Here's how the part is built. I have some questions about the finished solid (model axes, mm). Face numbers are marked on the shaded views. A direction names the side the tool comes from. Round coordinates to 2 decimals unless told otherwise and drop trailing zeros. Write each loop counter-clockwise with the first axis right and the second up, starting at its lowest first coordinate (ties: lowest second). Pieces come first, ordered by that corner, then holes. Notation, with made-up numbers: M -15.75,75.25 L 33.25,75.25 A27 cw 33.25,94.25 Z; hole C 88.25,49.25 d9. An arc over 180 degrees is marked long. Write item = value, one per line. Start each with the question number.
(1) I want a section at B-B (x = 58). List the corners of the cut face in (y, z) for me, and give its area (3 significant figures).
(2) I need wall thicknesses on line 1 along X through (y, z) = (30.75, 21); line 2 along Z through (x, y) = (20.5, 6.5); line 3 along X through (y, z) = (10, 23.5). Which ranges of each line are inside material? Lowest first, please.
(3) I want a section at D-D (x = 83). Give the number of separate pieces and of enclosed holes in the cut face, and give its area (3 significant figures).
(4) Will these pins go through, and if not, where does the flat tip stop? pin 1 Ø1 at (y, z) = (1.5, -35) entering from -X; pin 2 Ø5.5 at (x, y) = (86.5, 2.5) entering from +Z; pin 3 Ø1.5 at (x, z) = (84, -24) entering from +Y; pin 4 Ø4 at (x, y) = (28, 17.5) entering from -Z.
(5) I want a section at C-C (y = 21.5). List the corners of the cut face in (x, z) for me, and give its area (3 significant figures).
(6) I want a section at A-A (y = 8.5). List the corners of the cut face in (x, z) for me, and give its area (3 significant figures).
(7) On a 3-axis mill with a long thin cutter (end or side, diameter ignored), from which of +Z, -Z, +X, -X, +Y, -Y can I reach the whole of each face in a straight line? I mean the marked faces 4, 5 and 6. Say none if no direction works.
(8) If we mould it in two halves opening along X, with no side actions, what happens to the marked faces 1, 2 and 3? For each: released by +X, released by -X, zero draft, split by the parting line, or undercut.
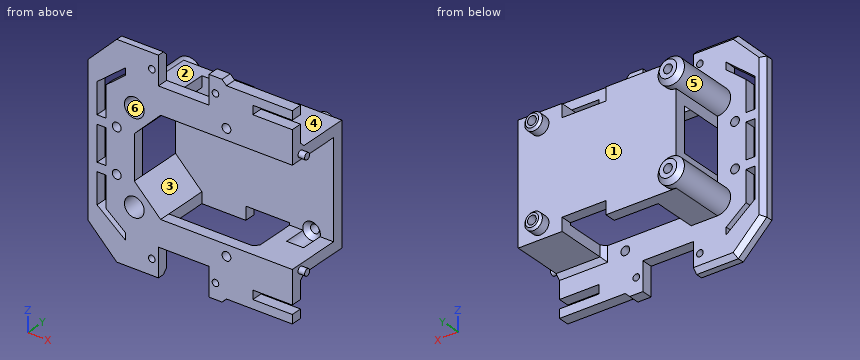
```python
from build123d import *

# Parameters (mm, degrees)
SKETCH1_R           = 2
SKETCH1_R_2         = 1.5
BOSS_EXTRUDE1_DEPTH = 5
SKETCH2_W           = 4
SKETCH2_H           = 16
CUT_EXTRUDE1_DEPTH  = 5
BOSS_EXTRUDE3_DEPTH = 25
SKETCH4_W           = 72
SKETCH4_H           = 54
BOSS_EXTRUDE4_DEPTH = 5
SKETCH5_W           = 40
SKETCH5_H           = 20
CUT_EXTRUDE2_DEPTH  = 123.576506721
SKETCH6_W           = 20
SKETCH6_H           = 6
CUT_EXTRUDE4_DEPTH  = 10
BOSS_EXTRUDE5_START = -5
SKETCH7_R           = 4
BOSS_EXTRUDE5_DEPTH = 5
SKETCH8_R           = 2
CUT_EXTRUDE5_DEPTH  = 10
CUT_EXTRUDE6_START  = 10
SKETCH9_R           = 4
CUT_EXTRUDE6_DEPTH  = 10
BOSS_EXTRUDE6_START = 5
SKETCH10_R          = 6
BOSS_EXTRUDE6_DEPTH = 30
SKETCH11_R          = 2
CUT_EXTRUDE7_DEPTH  = 10
CUT_EXTRUDE8_START  = 20
SKETCH12_R          = 4.5
CUT_EXTRUDE8_DEPTH  = 129.434311913
SKETCH14_R          = 4.5
CUT_EXTRUDE11_DEPTH = 108.158760724
SKETCH13_R          = 1.5
BOSS_EXTRUDE8_DEPTH = 3
CHAMFER2_SIZE       = 1
CHAMFER3_SIZE       = 2
CHAMFER4_SIZE       = 2
CHAMFER5_SIZE       = 2


with BuildPart() as part:
    # Sketch1 → Boss-Extrude1 (new body)
    with BuildSketch(Plane(origin=(0, 0, 0), x_dir=(1, 0, 0), z_dir=(0, 1, 0))):
        Polygon((0, 34), (0, -34), (13, -47), (32, -47), (32, -34), (55, -34), (55, -47), (61, -47), (63, -45), (93, -45), (93, -41), (75, -41), (75, -37), (93, -37), (93, -22), (33, -22), (21, -10), (21, 10), (33, 22), (93, 22), (93, 37), (75, 37), (75, 41), (93, 41), (93, 45), (63, 45), (61, 47), (55, 47), (55, 34), (32, 34), (32, 47), (13, 47), align=None)
        with Locations(Location((13, -10, 0), (0, 0, 270))):
            Circle(SKETCH1_R, mode=Mode.SUBTRACT)
        with Locations(Location((29, -40, 0), (0, 0, 270))):
            Circle(SKETCH1_R_2, mode=Mode.SUBTRACT)
        with Locations(Location((58, -40, 0), (0, 0, 270))):
            Circle(SKETCH1_R_2, mode=Mode.SUBTRACT)
        with Locations(Location((63, -27, 0), (0, 0, 270))):
            Circle(SKETCH1_R, mode=Mode.SUBTRACT)
        with Locations(Location((13, 10, 0), (0, 0, 90))):
            Circle(SKETCH1_R, mode=Mode.SUBTRACT)
        with Locations(Location((29, 40, 0), (0, 0, 90))):
            Circle(SKETCH1_R_2, mode=Mode.SUBTRACT)
        with Locations(Location((58, 40, 0), (0, 0, 90))):
            Circle(SKETCH1_R_2, mode=Mode.SUBTRACT)
        with Locations(Location((63, 27, 0), (0, 0, 90))):
            Circle(SKETCH1_R, mode=Mode.SUBTRACT)
    extrude(amount=BOSS_EXTRUDE1_DEPTH)

    # Sketch2 → Cut-Extrude1 (cut)
    with BuildSketch(Plane(origin=(0, 5, 0), x_dir=(1, 0, 0), z_dir=(0, 1, 0))):
        Polygon((17, 33.205766921), (17, 36.408329997), (4, 26), (4, 12), (8, 12), (8, 26), align=None)
        with Locations((6, 0)):
            Rectangle(SKETCH2_W, SKETCH2_H)
        Polygon((17, -33.205766921), (17, -36.408329997), (4, -26), (4, -12), (8, -12), (8, -26), align=None)
    extrude(amount=-CUT_EXTRUDE1_DEPTH, mode=Mode.SUBTRACT)

    # Sketch3 → Boss-Extrude3 (add)
    with BuildSketch(Plane(origin=(0, 5, 0), x_dir=(1, 0, 0), z_dir=(0, 1, 0))):
        Polygon((21, 27), (21, 10), (33, 22), (93, 22), (93, 27), align=None)
        Polygon((93, -27), (93, -22), (33, -22), (21, -10), (21, -27), align=None)
    extrude(amount=BOSS_EXTRUDE3_DEPTH)

    # Sketch4 → Boss-Extrude4 (add)
    with BuildSketch(Plane(origin=(0, 30, 0), x_dir=(1, 0, 0), z_dir=(0, 1, 0))):
        with Locations((57, 0)):
            Rectangle(SKETCH4_W, SKETCH4_H)
    extrude(amount=-BOSS_EXTRUDE4_DEPTH)

    # Sketch5 → Cut-Extrude2 (cut, through all)
    with BuildSketch(Plane.XY.offset(27)):
        with Locations((53, 15)):
            Rectangle(SKETCH5_W, SKETCH5_H)
    extrude(amount=-CUT_EXTRUDE2_DEPTH, mode=Mode.SUBTRACT)

    # Sketch6 → Cut-Extrude4 (cut)
    with BuildSketch(Plane(origin=(0, 30, 0), x_dir=(1, 0, 0), z_dir=(0, 1, 0))):
        with Locations((63, 24)):
            Rectangle(SKETCH6_W, SKETCH6_H)
        with Locations((63, -24)):
            Rectangle(SKETCH6_W, SKETCH6_H)
    extrude(amount=-CUT_EXTRUDE4_DEPTH, mode=Mode.SUBTRACT)

    # Sketch7 → Boss-Extrude5 (add)
    with BuildSketch(Plane.XZ.offset(-25).offset(BOSS_EXTRUDE5_START)):
        with Locations(Location((83, 21, 0), (0, 0, 270))):
            Circle(SKETCH7_R)
        with Locations(Location((83, -21, 0), (0, 0, 270))):
            Circle(SKETCH7_R)
    extrude(amount=-BOSS_EXTRUDE5_DEPTH)

    # Sketch8 → Cut-Extrude5 (cut)
    with BuildSketch(Plane(origin=(0, 35, 0), x_dir=(1, 0, 0), z_dir=(0, 1, 0))):
        with Locations(Location((83, 21, 0), (0, 0, 270))):
            Circle(SKETCH8_R)
    cut_extrude5 = extrude(amount=-CUT_EXTRUDE5_DEPTH, mode=Mode.SUBTRACT)

    # Sketch9 → Cut-Extrude6 (cut)
    with BuildSketch(Plane.XZ.offset(-25).offset(CUT_EXTRUDE6_START)):
        with Locations(Location((83, -21, 0), (0, 0, 270))):
            Circle(SKETCH9_R)
    cut_extrude6 = extrude(amount=-CUT_EXTRUDE6_DEPTH, mode=Mode.SUBTRACT)

    # Sketch10 → Boss-Extrude6 (add)
    with BuildSketch(Plane(origin=(0, 30, 0), x_dir=(1, 0, 0), z_dir=(0, 1, 0)).offset(BOSS_EXTRUDE6_START)):
        with Locations(Location((21, 21, 0), (0, 0, 270))):
            Circle(SKETCH10_R)
    boss_extrude6 = extrude(amount=-BOSS_EXTRUDE6_DEPTH)

    # Sketch11 → Cut-Extrude7 (cut)
    with BuildSketch(Plane(origin=(0, 35, 0), x_dir=(1, 0, 0), z_dir=(0, 1, 0))):
        with Locations(Location((21, 21, 0), (0, 0, 270))):
            Circle(SKETCH11_R)
    cut_extrude7 = extrude(amount=-CUT_EXTRUDE7_DEPTH, mode=Mode.SUBTRACT)

    # Sketch12 → Cut-Extrude8 (cut, through all)
    with BuildSketch(Plane(origin=(0, 5, 0), x_dir=(1, 0, 0), z_dir=(0, 1, 0)).offset(CUT_EXTRUDE8_START)):
        with Locations(Location((21, 21, 0), (0, 0, 270))):
            Circle(SKETCH12_R)
    extrude(amount=-CUT_EXTRUDE8_DEPTH, mode=Mode.SUBTRACT)

    # Mirror11: Cut-Extrude5, Cut-Extrude6 across plane
    add(cut_extrude5.mirror(Plane.XY), mode=Mode.SUBTRACT)
    add(cut_extrude6.mirror(Plane.XY), mode=Mode.SUBTRACT)

    # Mirror12: Boss-Extrude6 across plane
    add(boss_extrude6.mirror(Plane.XY))

    # Mirror16: Cut-Extrude7 across plane
    add(cut_extrude7.mirror(Plane.XY), mode=Mode.SUBTRACT)

    # Sketch14 → Cut-Extrude11 (cut, through all)
    with BuildSketch(Plane(origin=(0, 25, 0), x_dir=(1, 0, 0), z_dir=(0, 1, 0))):
        with Locations(Location((21, -21, 0), (0, 0, 270))):
            Circle(SKETCH14_R)
    extrude(amount=-CUT_EXTRUDE11_DEPTH, mode=Mode.SUBTRACT)

    # Sketch13 → Boss-Extrude8 (add)
    with BuildSketch(Plane(origin=(93, 0, 0), x_dir=(0, 0, -1), z_dir=(1, 0, 0))):
        with Locations(Location((24.5, 5, 0), (0, 0, 180))):
            Circle(SKETCH13_R)
    boss_extrude8 = extrude(amount=BOSS_EXTRUDE8_DEPTH)

    # Mirror19: Boss-Extrude8 across plane
    add(boss_extrude8.mirror(Plane.XY))

    # Chamfer2
    chamfer2_edges = [part.edges().sort_by_distance(p)[0] for p in [
        (83, 35, 25),
        (83, 35, -17),
    ]]
    chamfer(chamfer2_edges, length=CHAMFER2_SIZE)

    # Chamfer3
    chamfer3_edges = [part.edges().sort_by_distance(p)[0] for p in [
        (22.5, 5, -47),
        (6.5, 5, -40.5),
        (0, 5, 0),
        (6.5, 5, 40.5),
        (21, 35, -27),
        (21, 35, 27),
        (22.5, 5, 47),
    ]]
    chamfer(chamfer3_edges, length=CHAMFER3_SIZE)

    # Chamfer4
    chamfer4_edges = [part.edges().sort_by_distance(p)[0] for p in [
        (83, 5, -27),
        (83, 5, 27),
        (73, 5, 24.5),
        (73, 5, -24.5),
    ]]
    chamfer(chamfer4_edges, length=CHAMFER4_SIZE)

    # Chamfer5
    chamfer5_edges = [part.edges().sort_by_distance(p)[0] for p in [
        (83, 25, -23),
        (83, 25, 23),
    ]]
    chamfer(chamfer5_edges, length=CHAMFER5_SIZE - 0.0001)  # a hair under: the kernel refuses the full size


solid = part.part
```
Returned:
q1.outline = M 0,-47 L 5,-47 L 5,-41.5 L 0,-41.5 Z; M 0,-38.5 L 5,-38.5 L 5,-22 L 0,-22 Z; M 0,22 L 5,22 L 5,38.5 L 0,38.5 Z; M 0,41.5 L 5,41.5 L 5,47 L 0,47 Z; M 25,-21 L 30,-21 L 30,21 L 25,21 Z
q1.area = 430 mm²
q2.line_1 = 15 to 19, 23 to 27, 79 to 81, 85 to 87
q2.line_2 = -26.98 to -25.47, -16.53 to -15.02, 15.02 to 16.53, 25.47 to 26.98
q2.line_3 = 15.55 to 17.26, 24.74 to 33, 73 to 93
q3.separate_pieces = 5
q3.enclosed_holes = 0
q3.area = 594 mm²
q4.pin_1 = 0.5
q4.pin_2 = 45
q4.pin_3 = 35
q4.pin_4 = -27
q5.outline = M 21,-27 L 33,-27 L 33,-22 L 21,-10 L 21,-15 A6 ccw Z; M 21,10 L 33,22 L 33,27 L 21,27 A6 ccw 21,15 Z; M 73,-27 L 93,-27 L 93,-22 L 86.87,-22 A4 cw 79.13,-22 L 73,-22 Z; M 73,22 L 79.13,22 A4 cw 86.87,22 L 93,22 L 93,27 L 73,27 Z; hole C 21,-21 d9; hole C 21,21 d9
q5.area = 415 mm²
q6.outline = M 21,-27 L 33,-27 L 33,-22 L 21,-10 L 21,-15 A6 ccw Z; M 21,10 L 33,22 L 33,27 L 21,27 A6 ccw 21,15 Z; M 73,-27 L 93,-27 L 93,-22 L 73,-22 Z; M 73,22 L 93,22 L 93,27 L 73,27 Z; hole C 21,-21 d9; hole C 21,21 d9
q6.area = 450 mm²
q7.face_4 = +Z, +X, -X, +Y
q7.face_5 = +Y
q7.face_6 = -Y
q8.face_1 = undercut
q8.face_2 = zero draft
q8.face_3 = released by +X
